Build history of the part. All positions in model axes, mm. A direction names the side the tool comes from. Round coordinates to 2 decimals unless told otherwise and drop trailing zeros. Loops run counter-clockwise (first coordinate to the right, second up) from the corner with the lowest first, then second, coordinate; pieces in that order, holes last.
from build123d import *

# Parameters (mm, degrees)
SKETCH_4_W             = 255
SKETCH_4_H             = 250
EXTRUDE_2_DEPTH        = 10
SKETCH_7_W             = 20
SKETCH_7_H             = 250
EXTRUDE_3_DEPTH        = 90
EXTRUDE_4_DEPTH        = 30
CUT_EXTRUDE_1_REACH    = 303.081
SKETCH_9_R             = 10
SKETCH_11_W            = 60
SKETCH_11_H            = 10
EXTRUDE_6_DEPTH        = 5
FILLET_1_R             = 5
FILLET_1_OF_MIRROR_2_R = 5


with BuildPart() as part:
    # 草圖4 → 填料-伸長2 (new body)
    with BuildSketch(Plane(origin=(0, 0, 0), x_dir=(1, 0, 0), z_dir=(0, 1, 0))):
        Rectangle(SKETCH_4_W, SKETCH_4_H)
    extrude(amount=EXTRUDE_2_DEPTH)

    # 草圖7 → 填料-伸長3 (add)
    with BuildSketch(Plane(origin=(0, 10, 0), x_dir=(1, 0, 0), z_dir=(0, 1, 0))):
        with Locations((-117.5, 0)):
            Rectangle(SKETCH_7_W, SKETCH_7_H)
        with Locations((117.5, 0)):
            Rectangle(SKETCH_7_W, SKETCH_7_H)
    extrude(amount=EXTRUDE_3_DEPTH)

    # 草圖8 → 填料-伸長4 (add)
    with BuildSketch(Plane.XY.offset(125)):
        Polygon((-30, 10), (-38, 10), (-38, 55), (-30, 55), (-30, 45), (30, 45), (30, 55), (38, 55), (38, 10), (30, 10), (30, 40), (-30, 40), align=None)
    extrude_4 = extrude(amount=-EXTRUDE_4_DEPTH)

    # 草圖9 → 除料-伸長1 (cut, up to next)
    with BuildSketch(Plane.ZY.offset(127.5), mode=Mode.PRIVATE) as cut_extrude_1_sk1:
        with Locations((-25, 25)):
            Circle(SKETCH_9_R)
    cut_extrude_1_tool1 = extrude(cut_extrude_1_sk1.sketch, amount=-CUT_EXTRUDE_1_REACH, mode=Mode.PRIVATE) & part.part
    cut_extrude_1 = cut_extrude_1_tool1.solids().sort_by_distance((-127.5, 25, -25))[0]
    add(cut_extrude_1, mode=Mode.SUBTRACT)

    # 鏡射1: 除料-伸長1 across plane
    add(cut_extrude_1.mirror(Plane(origin=(0, 0, 0), x_dir=(0, 0, 1), z_dir=(1, 0, 0))), mode=Mode.SUBTRACT)

    # 草圖11 → 填料-伸長6 (add)
    with BuildSketch(Plane.XY.offset(125)):
        with Locations((0, 50)):
            Rectangle(SKETCH_11_W, SKETCH_11_H)
    extrude_6 = extrude(amount=-EXTRUDE_6_DEPTH)

    # 圓角1
    fillet_1_edges = [part.edges().sort_by_distance(p)[0] for p in [
        (-34, 10, 95),
        (-30, 10, 110),
        (-38, 10, 110),
        (34, 10, 95),
        (38, 10, 110),
        (30, 10, 110),
    ]]
    fillet(fillet_1_edges, radius=FILLET_1_R)

    # 鏡射2: 填料-伸長4, 填料-伸長6 across plane
    add(extrude_4.mirror(Plane(origin=(0, 0, 30), x_dir=(1, 0, 0), z_dir=(0, 0, -1))))
    add(extrude_6.mirror(Plane(origin=(0, 0, 30), x_dir=(1, 0, 0), z_dir=(0, 0, -1))))

    # 圓角1 of 鏡射2
    fillet_1_of_mirror_2_edges = [part.edges().sort_by_distance(p)[0] for p in [
        (-34, 10, -35),
        (-30, 10, -50),
        (-38, 10, -50),
        (34, 10, -35),
        (38, 10, -50),
        (30, 10, -50),
    ]]
    fillet(fillet_1_of_mirror_2_edges, radius=FILLET_1_OF_MIRROR_2_R)


solid = part.part
(1) Pin check, flat tips, straight feed: P1, Ø15, axis at x = 11.5, z = 112, coming from the -Y side; P2, Ø2, axis at x = -74, z = 13.5, coming from the +Y side; P3, Ø11, axis at x = 4.5, y = 52.5, coming from the -Z side. Stop position of each tip, or through.
Responses:
P1: stops at y = 0
P2: stops at y = 10
P3: stops at z = -65
(2) Probe line 1 (X direction, y = 36, z = -37); line 2 (X direction, y = 81.5, z = 95.5); line 3 (Y direction, x = 123, z = -25). List the from-to ranges inside material, lowest first.
Responses:
line 1: x = -127.5 to -107.5, -38 to -30, 30 to 38, 107.5 to 127.5
line 2: x = -127.5 to -107.5, 107.5 to 127.5
line 3: y = 0 to 15, 35 to 100
(3) Slice it at C-C on x = -9.5. List the corners of the cut face in (y, z), plus the area to 3 significant figures.
Responses:
outline: (0, -125) - (10, -125) - (10, 125) - (0, 125) - close; (40, -65) - (55, -65) - (55, -60) - (45, -60) - (45, -35) - (40, -35) - close; (40, 95) - (45, 95) - (45, 120) - (55, 120) - (55, 125) - (40, 125) - close
area: 2,900 mm2
(4) Slice it at B-B on z = -25. List the corners of the cut face in (x, y), plus the area to 3 significant figures.
Responses:
outline: (-127.5, 0) - (127.5, 0) - (127.5, 15) - (107.5, 15) - (107.5, 10) - (-107.5, 10) - (-107.5, 15) - (-127.5, 15) - close; (-127.5, 35) - (-107.5, 35) - (-107.5, 100) - (-127.5, 100) - close; (107.5, 35) - (127.5, 35) - (127.5, 100) - (107.5, 100) - close
area: 5,350 mm2
(5) Pull direction Z, two halves, no side cores. Call faces 5 (the face through (38, 35, 110)), 6 (the face through (-1, 9, -125)), 7 (the face through (-30, 50, 108)): +Z half, -Z half, draft (parallel to the pull), parting line (faces both ways), or undercut.
Responses:
face 5: draft
face 6: -Z half
face 7: undercut
(6) Which spindle directions (+Z, -Z, +X, -X, +Y, -Y) get a long thin tool onto all of the face, cutting with end or side? Do faces 1 (the face through (-2, 51, 125)), 2 (the face through (-30, 28, -50)), 3 (the face through (107.5, 54, 2)), 4 (the face through (3, 41, 95)). Say none if no direction does.
Responses:
face 1: +Z, +X, -X, +Y, -Y
face 2: +Z, -Z
face 3: +Z, -Z, +Y
face 4: +Y
(7) Slice it at A-A on y = 25. Count the separate pieces of the cut face and the enclosed holes in it, plus the area to 3 significant figures.
Responses:
separate pieces: 8
enclosed holes: 0
area: 10,200 mm2
(8) Slice it at D-D on z = -55.5. List the corners of the cut face in (x, y).
Responses:
outline: (-127.5, 0) - (127.5, 0) - (127.5, 100) - (107.5, 100) - (107.5, 10) - (43, 10) arc R5 cw to (38, 15) - (38, 55) - (30, 55) - (30, 45) - (-30, 45) - (-30, 55) - (-38, 55) - (-38, 15) arc R5 cw to (-43, 10) - (-107.5, 10) - (-107.5, 100) - (-127.5, 100) - close; hole (-30, 15) arc R5 ccw to (-25, 10) - (25, 10) arc R5 ccw to (30, 15) - (30, 40) - (-30, 40) - close
